Work out the finished part from the listing and answer in its coordinate system (mm). Face numbers are marked on the shaded views. A direction names the side the tool comes from. Coordinates: 2 decimals unless noted, no trailing zeros. Loops run counter-clockwise (first coordinate to the right, second up) from the corner with the lowest first, then second, coordinate; pieces in that order, holes last. Notation, with made-up numbers: (2.5, 17) - (6.5, 17) arc R28 cw to (6.5, 49) - close; hole circle Ø3 at (72.5, 20). An arc over 180 degrees is marked (long way). Write each question's results on one line, items separated by ' | '. Start each with the question number.
Item 1: Consider probe 1 along X at (y, z) = (0, 0.35); probe 2 along Y at (x, z) = (0, 0.2). Determine where each line is inside the solid, lowest interval first. Write a range as [from, to].
Item 2: Section B-B, the plane z = 1.3 is taken. Write down the section's boundary in (x, y), plus the area to 3 significant figures.
Item 3: For a pull along Y with two mould halves and no side action, classify the marked faces 6, 7 and 8 as +Y half, -Y half, draft (parallel to the pull), parting line (faces both ways), or undercut.
Item 4: A tool of negligible diameter and unlimited length cuts with its end or side. For the marked faces 1, 2, 3, 4 and 5, from which of +Z, -Z, +X, -X, +Y, -Y can it reach the whole face along a straight path? Write none if from no direction.
Item 5: Section A-A, the plane x = 3.25 is taken. Write down the section's boundary in (y, z), plus the area to 3 significant figures.
Item 6: Each of these flat-tipped pins is pushed along its axis until it touches: pin 1 Ø2 at (x, z) = (-1.5, 1) entering from +Y; pin 2 Ø0.8 at (x, y) = (3.5, 0.5) entering from +Z; pin 3 Ø1 at (y, z) = (-0.5, 4) entering from -X. Where does it stop, or does it pass through?
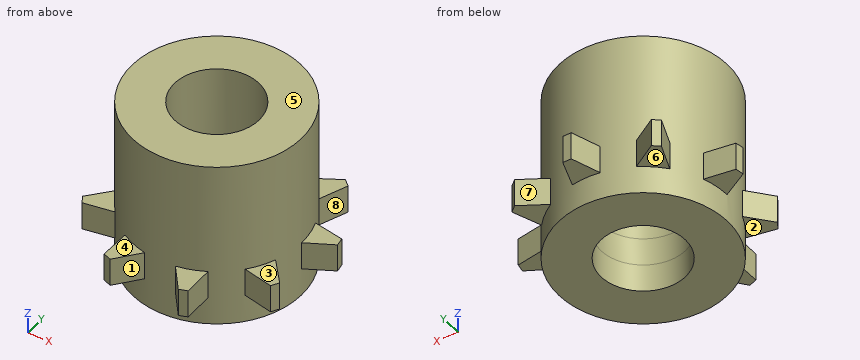
Autodesk Inventor part; units mm, degrees
ref_plane "YZ Plane" through (0, 0, 0) normal (1, 0, 0) x (0, 1, 0)
ref_plane "XZ Plane" through (0, 0, 0) normal (0, 1, 0) x (-1, 0, 0)
ref_plane "XY Plane" through (0, 0, 0) normal (0, 0, 1) x (1, 0, 0)
sketch "Sketch1" plane through (0, 0, 0) normal (0, 0, 1) x (1, 0, 0)
  circle A0 centre (0, 0) radius 3
  circle A1 centre (0, 0) radius 1.5
  dimension "d0" = 6
  dimension "d1" = 3
extrude "Extrusion1" add sketch "Sketch1" along normal blind 1
sketch "Sketch3" plane through (0, 0, 0) normal (0, 0, -1) x (-1, 0, 0)
  circle A0 centre (0, 0) radius 1.5
  circle A1 centre (0, 0) radius 3
extrude "Extrusion3" add sketch "Sketch3" along normal blind 1
sketch "Sketch2" plane through (0, 0, 1) normal (0, 0, 1) x (1, 0, 0)
  line L0 (0, 0) -> (0, 3.959) construction
  line L1 (-0.15, 3.959) -> (0.15, 3.959)
  line L2 (-0.4943, 2.959) -> (0.4943, 2.959)
  line L3 (-0.15, 3.959) -> (-0.4943, 2.959)
  line L4 (0.15, 3.959) -> (0.4943, 2.959)
  circle A0 centre (0, 0) radius 3
  point P0 (0, 2.959)
  dimension "d4" = 1
  dimension "d5" = 0.3
  dimension "d8" = 109
extrude "Extrusion2" add sketch "Sketch2" against normal up to surface (1 mm away) separate body contours L1 L4 A0 L3 | A0 L2 picked at (-0.0551, 2.9711)
sketch "Sketch4" plane through (0, 0, 1) normal (0, 0, 1) x (1, 0, 0)
  circle A0 centre (0, 0) radius 1.5
  circle A1 centre (0, 0) radius 3
extrude "Extrusion4" add sketch "Sketch4" along normal blind 4 bodies 1
pattern_circular "Circular Pattern1" count 9 over 360 about axis through (0, 0, 0) along (0, 0, 1) of "Extrusion2" bodies 2
combine bodies "Combine1" operation type add bodies to combine 1 2
properties part number "ChainGear"
Answer key:
1) probe 1: x = [-3, -1.5], [1.5, 3] | probe 2: y = [-3, -1.5], [1.5, 3.96]
2) outline: circle Ø6 at (0, 0); hole circle Ø3 at (0, 0) | area: 21.2 mm^2
3) face 6: draft | face 7: +Y half | face 8: undercut
4) face 1: +Z, -Z, -Y | face 2: -Z, -X, -Y | face 3: +Z, +X, -Y | face 4: +Z, -X, -Y | face 5: +Z, +X, -X, +Y, -Y
5) outline: (-2.09, 0) - (-1.56, 0) - (-1.56, 1) - (-2.09, 1) - close; (0.17, 0) - (0.93, 0) - (0.93, 1) - (0.17, 1) - close | area: 1.30 mm^2
6) pin 1: stops at y = 3.13 | pin 2: stops at z = 1 | pin 3: stops at x = -3
